from build123d import *

# Parameters (mm, degrees)
BOSS_EXTRUDE1_DEPTH     = 10
CUT_EXTRUDE2_DEPTH      = 25
SKETCH4_W               = 2.420711262391846
SKETCH4_H               = 16.924538398432034
CUT_EXTRUDE3_DEPTH      = 25
CUT_EXTRUDE4_DEPTH      = 15.000000000000002
FILLET1_R               = 4
SKETCH6_R               = 3
BOSS_EXTRUDE2_DEPTH     = 1
SKETCH7_W               = 9.06468295299787
SKETCH7_H               = 3
CUT_EXTRUDE5_DEPTH      = 1.5
FILLET2_R               = 1
SKETCH8_R               = 1.500000000000004
BOSS_EXTRUDE3_DEPTH     = 1.75
CUT_EXTRUDE7_DEPTH      = 47.435439052516784
CUT_EXTRUDE7_DEPTH_BACK = 47.435439052516784
SKETCH9_R               = 1
SKETCH10_R              = 2.4999999999999982
CUT_EXTRUDE8_DEPTH      = 47.435439052516784


with BuildPart() as part:
    # Sketch1 → Boss-Extrude1 (new, symmetric)
    with BuildSketch(Plane.XY):
        Polygon((34.99999999999999, -12.5), (-35.00000000000001, -12.500000000000005), (-35.00000000000001, 12.499999999999995), (34.99999999999999, 12.500000000000002), align=None)
    extrude(amount=BOSS_EXTRUDE1_DEPTH, both=True)

    # Sketch2 → Cut-Extrude2 (cut)
    with BuildSketch(Plane(origin=(34.99999999999999, 0, 0), x_dir=(0, 0, -1), z_dir=(1, 0, 0))):
        with BuildLine():
            Line((-10, 12.500000000000002), (-10, 7.500000000000002))
            ThreePointArc((-9.999999999999998, 7.500000000000003), (-5.590169943749482, 11.180339887498945), (-1.821e-14, 12.500000000000004))
            Line((-1.776e-14, 12.500000000000002), (-10, 12.500000000000002))
        make_face()
        with BuildLine():
            Line((10, 12.500000000000002), (-1.776e-14, 12.500000000000002))
            ThreePointArc((-1.821e-14, 12.500000000000004), (5.590169943749467, 11.180339887498956), (10, 7.500000000000001))
            Line((10, 7.500000000000002), (10, 12.500000000000002))
        make_face()
        with BuildLine():
            ThreePointArc((9.999999999999998, -7.500000000000003), (5.590169943749469, -11.180339887498953), (-1.554e-14, -12.5))
            Line((-1.599e-14, -12.5), (10, -12.5))
            Line((10, -12.5), (10, -7.500000000000002))
        make_face()
        with BuildLine():
            ThreePointArc((-1.554e-14, -12.5), (-5.590169943749482, -11.180339887498945), (-10, -7.500000000000001))
            Line((-10, -7.500000000000002), (-10, -12.5))
            Line((-10, -12.5), (-1.599e-14, -12.5))
        make_face()
    extrude(amount=-CUT_EXTRUDE2_DEPTH, mode=Mode.SUBTRACT)

    # Sketch4 → Cut-Extrude3 (cut)
    with BuildSketch(Plane(origin=(34.99999999999999, 0, 0), x_dir=(0, 0, -1), z_dir=(1, 0, 0))):
        with Locations((-10.41035563119592, 0)):
            Rectangle(SKETCH4_W, SKETCH4_H)
    extrude(amount=-CUT_EXTRUDE3_DEPTH, mode=Mode.SUBTRACT)

    # Sketch5 → Cut-Extrude4 (cut)
    with BuildSketch(Plane(origin=(34.99999999999999, 0, 0), x_dir=(0, 0, -1), z_dir=(1, 0, 0))):
        with BuildLine():
            Line((-9.199999999999998, 8.462269199216015), (-9.199999999999996, -8.462269199216017))
            ThreePointArc((-9.199999999999996, -8.462269199216017), (0.6256920192394629, -12.484330558626684), (10, -7.500000000000002))
            Line((10, -7.500000000000002), (10, 7.500000000000002))
            ThreePointArc((10, 7.500000000000002), (0.6256920192394629, 12.484330558626686), (-9.199999999999998, 8.462269199216015))
        make_face()
        with BuildLine():
            Line((-8.399999999999997, 8.144323176298942), (-8.399999999999997, -8.144323176298942))
            ThreePointArc((-8.399999999999997, -8.144323176298942), (0.608047219709459, -11.684189256367068), (9.2, -7.228416147400481))
            Line((9.2, -7.228416147400481), (9.2, 7.228416147400481))
            ThreePointArc((9.2, 7.228416147400481), (0.6080472197094615, 11.684189256367066), (-8.399999999999997, 8.144323176298942))
        make_face(mode=Mode.SUBTRACT)
    extrude(amount=-CUT_EXTRUDE4_DEPTH, mode=Mode.SUBTRACT)

    # Fillet1
    # the kernel refuses this fillet: 4 mm, written as the material it takes off along each edge
    with BuildSketch(Plane(origin=(34.99999999999999, -4.44e-15, 6.7e-16), x_dir=(0, -0.1880210929197643, -0.982164990527181), z_dir=(0, -0.982164990527181, 0.1880210929197643))) as fillet1_piece_1:
        with BuildLine():
            CenterArc((11.700000000000003 - FILLET1_R, -FILLET1_R), FILLET1_R, 0, 89.99999999999999)
            Line((11.700000000000003 - FILLET1_R, 0), (11.700000000000003, 0))
            Line((11.700000000000003, 0), (11.700000000000003, -FILLET1_R))
        make_face()
    revolve(axis=Axis((34.99999999999999, -4.44e-15, 6.7e-16), (1, 0, 0)), revolution_arc=195.71664993769073, mode=Mode.SUBTRACT)
    with BuildSketch(Plane(origin=(34.99999999999999, -17.22841614740048, -9.2), x_dir=(-1, 0, 0), z_dir=(0, 1, 0))) as fillet1_piece_2:
        with BuildLine():
            CenterArc((FILLET1_R, FILLET1_R), FILLET1_R, 180, 90)
            Line((0, FILLET1_R), (0, 0))
            Line((0, 0), (FILLET1_R, 0))
        make_face()
    extrude(amount=34.45683229480096, mode=Mode.SUBTRACT)
    with BuildSketch(Plane(origin=(34.99999999999999, 0, 6.7e-16), x_dir=(0, 0.0850574768635666, 0.9963760462945724), z_dir=(0, 0.9963760462945724, -0.0850574768635666))) as fillet1_piece_3:
        with BuildLine():
            CenterArc((11.700000000000003 - FILLET1_R, -FILLET1_R), FILLET1_R, 0, 90)
            Line((11.700000000000003 - FILLET1_R, 0), (11.700000000000003, 0))
            Line((11.700000000000003, 0), (11.700000000000003, -FILLET1_R))
        make_face()
    revolve(axis=Axis((34.99999999999999, 0, 6.7e-16), (1, 0, 0)), revolution_arc=195.71664993769085, mode=Mode.SUBTRACT)
    with BuildSketch(Plane(origin=(34.99999999999999, 18.14432317629894, 8.399999999999997), x_dir=(-1, 0, 0), z_dir=(0, -1, 0))) as fillet1_piece_4:
        with BuildLine():
            CenterArc((FILLET1_R, FILLET1_R), FILLET1_R, 180, 90)
            Line((0, FILLET1_R), (0, 0))
            Line((0, 0), (FILLET1_R, 0))
        make_face()
    extrude(amount=36.28864635259788, mode=Mode.SUBTRACT)

    # Sketch6 → Boss-Extrude2 (add)
    with BuildSketch(Plane(origin=(34.99999999999999, 0, 0), x_dir=(0, 0, -1), z_dir=(1, 0, 0))):
        with Locations(Location((0, 0, 0), (0, 0, 180))):
            Circle(SKETCH6_R)
    extrude(amount=BOSS_EXTRUDE2_DEPTH)

    # Sketch7 → Cut-Extrude5 (cut)
    with BuildSketch(Plane(origin=(0, 0, -9.2), x_dir=(-1, 0, 0), z_dir=(0, 0, -1))):
        with Locations((-27.832741428017933, 0)):
            Rectangle(SKETCH7_W, SKETCH7_H)
    cut_extrude5 = extrude(amount=-CUT_EXTRUDE5_DEPTH, mode=Mode.SUBTRACT)

    # Mirror1: Cut-Extrude5 across plane
    add(cut_extrude5.mirror(Plane.XY), mode=Mode.SUBTRACT)

    # Fillet2
    fillet2_edges = [part.edges().sort_by_distance(p)[0] for p in [
        (-35.00000000000001, 12.499999999999995, 0),
        (-35.00000000000001, -12.500000000000005, 0),
    ]]
    fillet(fillet2_edges, radius=FILLET2_R)

    # Sketch8 → Boss-Extrude3 (add, symmetric)
    with BuildSketch(Plane.XY):
        Polygon((-35.00000000000001, -2.4999999999999987), (-40.00000000000001, -2.499999999999998), (-40.00000000000001, 2.500000000000002), (-35.00000000000001, 2.4999999999999987), align=None)
        with Locations((-37.50000000000001, 2.17e-15)):
            Circle(SKETCH8_R, mode=Mode.SUBTRACT)
    extrude(amount=BOSS_EXTRUDE3_DEPTH, both=True)

    # Sketch9 → Cut-Extrude7 (cut, two sides: drawn at the far end of the back side and taken through both)
    with BuildSketch(Plane.XY.offset(10).offset(-CUT_EXTRUDE7_DEPTH_BACK)):
        with Locations(Location((4.99999999999999, -10.500000000000004, 0), (0, 0, 180))):
            Circle(SKETCH9_R)
        with Locations(Location((4.99999999999999, 10.500000000000004, 0), (0, 0, 180))):
            Circle(SKETCH9_R)
    extrude(amount=CUT_EXTRUDE7_DEPTH + CUT_EXTRUDE7_DEPTH_BACK, mode=Mode.SUBTRACT)

    # Sketch10 → Cut-Extrude8 (cut, through all)
    with BuildSketch(Plane(origin=(0, 0, -10), x_dir=(-1, 0, 0), z_dir=(0, 0, -1))):
        with Locations((23.00000000000001, 0)):
            Circle(SKETCH10_R)
    extrude(amount=-CUT_EXTRUDE8_DEPTH, mode=Mode.SUBTRACT)


solid = part.part
The listing builds one solid part. Answer for the finished solid, in the listing's coordinates (mm). A direction names the side the tool comes from. Coordinates: 2 decimals unless noted, no trailing zeros. Loops run counter-clockwise (first coordinate to the right, second up) from the corner with the lowest first, then second, coordinate; pieces in that order, holes last. Notation, with made-up numbers: (84.5, -12) -> (92.5, -12) arc R25 ccw to (92.5, 3) -> close; hole circle Ø9 at (-4.5, -37.75). An arc over 180 degrees is marked (long way). Answer in a Markdown table with one row per item. Add a question column.
1. Consider line 1 (Y direction, x = 5, z = -3); line 2 (Y direction, x = -37.5, z = 0.3); line 3 (Z direction, x = 26.5, y = -7.25). Determine where each line is inside the solid, lowest interval first. Write a range as [from, to].
2. The part is cut by section A-A, the plane x = -23. Write down the section's boundary in (y, z), then the cut area to 3 significant figures.
3. Determine the mould class of faces 6 (the flat face through (36, 0, 0)), 7 (the cylindrical face through (25.577, 11.676, -0.748)), 8 (the flat face through (28, -1.5, -8)) for opening direction Y: +Y half, -Y half, draft (parallel to the pull), parting line (faces both ways), or undercut.
4. The part is cut by section B-B, the plane y = 0. Count the separate pieces of the cut face and the enclosed holes in it, then the cut area to 3 significant figures.
5. For faces 1 (the flat face through (23.3, 0, -8)), 2 (the flat face through (10, 0.1, 9.5)), 3 (the flat face through (10, -11, -8)), 4 (the flat face through (-37, -2.5, 0)), 5 (the cylindrical face through (15.07, 12.49, -0.47)), determine the directions among +Z, -Z, +X, -X, +Y, -Y from which every point of the face is accessible in a straight line to the end or side of a thin tool.
6. The part is cut by section C-C, the plane x = 5. Write down the section's boundary in (y, z), then the cut area to 3 significant figures.
7. The part is cut by section D-D, the plane x = 28. Write down the section's boundary in (y, z), then the cut area to 3 significant figures.
8. Flat-ended cylindrical pins translate along their axes: P1, Ø2, axis at y = 3, z = 5.5, coming from the -X side; P2, Ø5, axis at y = 4.5, z = 5, coming from the +X side; P3, Ø0.9, axis at x = 30, y = 0, coming from the -Z side. Find the tip coordinate at first contact, or state that the pin passes through.
Answer below:
| question | item | result |
|---|---|---|
| 1 | line 1 | [-12.5, -11.5], [-9.5, 9.5], [11.5, 12.5] |
| 1 | line 2 | [-2.5, -1.5], [1.5, 2.5] |
| 1 | line 3 | [-9.18, 8.4] |
| 2 | outline | (-12.5, -10) -> (-2.5, -10) -> (-2.5, 10) -> (-12.5, 10) -> close; (2.5, -10) -> (12.5, -10) -> (12.5, 10) -> (2.5, 10) -> close |
| 2 | area | 400 mm2 |
| 3 | face 6 | draft |
| 3 | face 7 | +Y half |
| 3 | face 8 | undercut |
| 4 | separate pieces | 3 |
| 4 | enclosed holes | 0 |
| 4 | area | 1,240 mm2 |
| 5 | face 1 | -Z |
| 5 | face 2 | +Z, +X |
| 5 | face 3 | -Z, +X, -Y |
| 5 | face 4 | +Z, -Z, -X, -Y |
| 5 | face 5 | +X, +Y |
| 6 | outline | (-12.5, -10) -> (-11.5, -10) -> (-11.5, 10) -> (-12.5, 10) -> close; (-9.5, -10) -> (9.5, -10) -> (9.5, 10) -> (-9.5, 10) -> close; (11.5, -10) -> (12.5, -10) -> (12.5, 10) -> (11.5, 10) -> close |
| 6 | area | 420 mm2 |
| 7 | outline | (-8.14, 8.4) arc R11.7 ccw to (-7.23, -9.2) -> (-1.5, -9.2) -> (-1.5, -7.7) -> (1.5, -7.7) -> (1.5, -9.2) -> (7.23, -9.2) arc R11.7 ccw to (8.14, 8.4) -> (1.5, 8.4) -> (1.5, 7.7) -> (-1.5, 7.7) -> (-1.5, 8.4) -> close |
| 7 | area | 362 mm2 |
| 8 | P1 | x = -35 |
| 8 | P2 | x = 35 |
| 8 | P3 | z = -7.7 |
